Design review of the part shown in the three views and the two pictorial views. Dimensions are in mm from the part's minimum x, y and z. A direction names the side the tool comes from. Give positions to 0.01 mm unless a question says otherwise; leave off trailing zeros. Loops run counter-clockwise (first coordinate to the right, second up) from the corner with the lowest first, then second, coordinate; pieces in that order, holes last. Notation, with made-up numbers: (-6.5, 45.5) -> (2.5, 45.5) arc R19 ccw to (2.5, 63.5) -> close; hole circle Ø1 at (7.25, -26.75). An arc over 180 degrees is marked (long way). Answer as CSV lines item,"result". Start each with the question number.
Item 1: For L1, parallel to X at y = 10.5, z = 19; L2, parallel to X at y = 0.4, z = 13.5; L3, parallel to Z at x = 8.5, y = 6.5, list the stretches that pass through material, from the lowest coordinate up. Write a range as from..to.
Item 2: Add section A-A on x = 17.5. State the section outline as (y, z) points, plus the area to 3 significant figures.
Item 3: The part is to be moulded in two halves that separate along Z. For the marked faces 3, 4 and 5, say which applies: +Z half, -Z half, draft (parallel to the pull), parting line (faces both ways), or undercut.
Item 4: Add section B-B on z = 13.5. State the section outline as (x, y) points, plus the area to 3 significant figures.
Item 5: Add section C-C on y = 4. State the section outline as (x, z) points, plus the area to 3 significant figures.
Item 6: Clearance check with flat-ended pins moving along their axes: P1, Ø10, axis at x = 11.5, z = 12.5, coming from the -Y side; P2, Ø6, axis at y = 8, z = 7, coming from the -X side. State where each tip first meets the part, or that it passes through.
Item 7: Machinability: for the marked faces 1 and 2, which of the approach directions +Z, -Z, +X, -X, +Y, -Y give a long, thin tool a straight path to every point of the face, cutting with its end or side? Answer none if there is none.
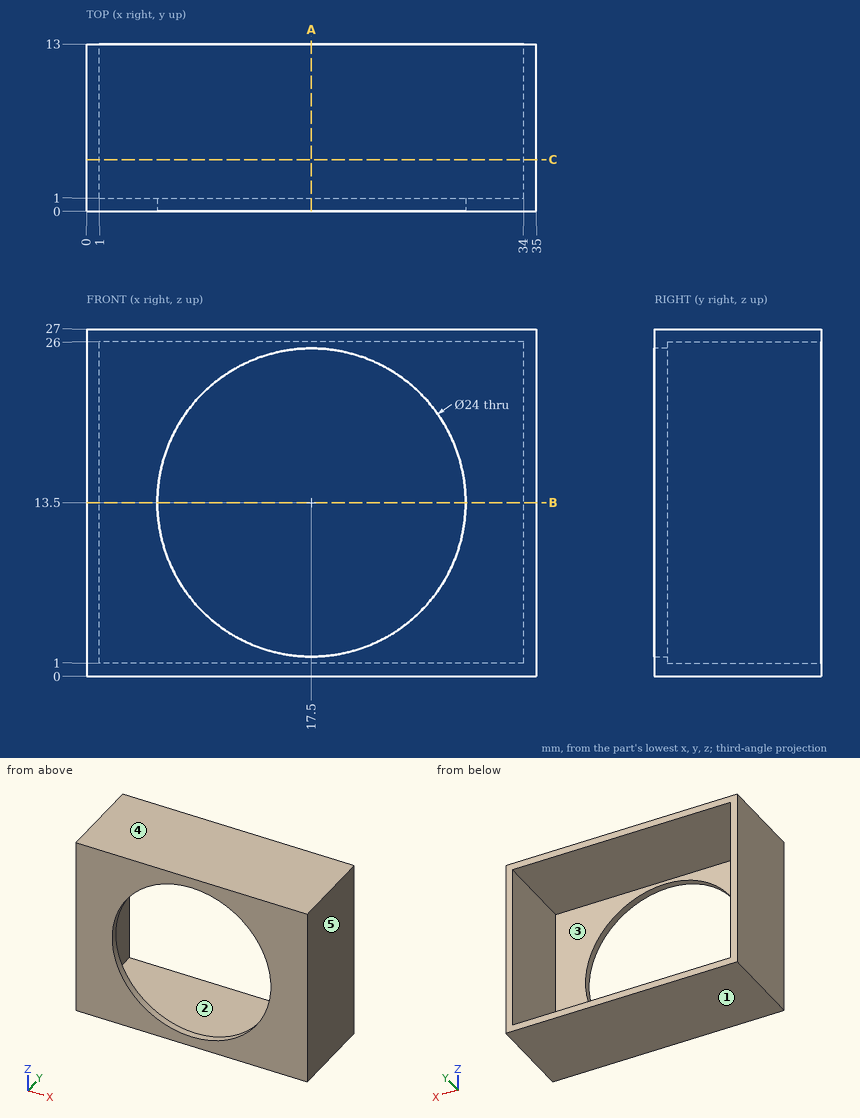
Computed values:
1,L1,"0..1, 34..35"
1,L2,"0..5.5, 29.5..35"
1,L3,"0..1, 26..27"
2,outline,"(0, 0) -> (13, 0) -> (13, 1) -> (1, 1) -> (1, 1.5) -> (0, 1.5) -> close; (0, 25.5) -> (1, 25.5) -> (1, 26) -> (13, 26) -> (13, 27) -> (0, 27) -> close"
2,area,"27.0 mm²"
3,face 3,"undercut"
3,face 4,"+Z half"
3,face 5,"draft"
4,outline,"(0, 0) -> (5.5, 0) -> (5.5, 1) -> (1, 1) -> (1, 13) -> (0, 13) -> close; (29.5, 0) -> (35, 0) -> (35, 13) -> (34, 13) -> (34, 1) -> (29.5, 1) -> close"
4,area,"35.0 mm²"
5,outline,"(0, 0) -> (35, 0) -> (35, 27) -> (0, 27) -> close; hole (1, 1) -> (34, 1) -> (34, 26) -> (1, 26) -> close"
5,area,"120 mm²"
6,P1,"through"
6,P2,"x = 0"
7,face 1,"-Z, +X, -X, +Y, -Y"
7,face 2,"+Y"
